```python
from build123d import *

# Parameters (mm, degrees)
CROQUIS1_R              = 1.75
SALIENTE_EXTRUIR1_DEPTH = 3


with BuildPart() as part:
    # Croquis1 → Saliente-Extruir1 (new body)
    with BuildSketch(Plane.XY):
        with BuildLine():
            Line((13.871153062, 23.274726508), (24.330135763, 23.274726508))
            ThreePointArc((24.330135763, 23.274726508), (24.799781514, 23.311715731), (25.257846044, 23.421771263))
            Line((25.257846044, 23.421771263), (32.405644412, 25.746057998))
            ThreePointArc((32.405644412, 25.746057998), (34.336780797, 30.811489821), (28.935644412, 30.347148308))
            Line((28.935644412, 30.347148308), (23.249258293, 28.345004197))
            ThreePointArc((23.249258293, 28.345004197), (22.758316719, 28.21760232), (22.252929212, 28.174726508))
            Line((22.252929212, 28.174726508), (15.948359613, 28.174726508))
            ThreePointArc((15.948359613, 28.174726508), (15.442972106, 28.21760232), (14.952030531, 28.345004197))
            Line((14.952030531, 28.345004197), (9.265644412, 30.347148308))
            ThreePointArc((9.265644412, 30.347148308), (3.864508027, 30.811489821), (5.795644412, 25.746057998))
            Line((5.795644412, 25.746057998), (12.94344278, 23.421771263))
            ThreePointArc((12.94344278, 23.421771263), (13.401507311, 23.311715731), (13.871153062, 23.274726508))
        make_face()
        with Locations((31.781902577, 28.88467969)):
            Circle(CROQUIS1_R, mode=Mode.SUBTRACT)
        with Locations(Location((6.419386247, 28.88467969, 0), (0, 0, 180))):
            Circle(CROQUIS1_R, mode=Mode.SUBTRACT)
    extrude(amount=SALIENTE_EXTRUIR1_DEPTH)


solid = part.part
```
The listing builds one solid part. Answer for the finished solid, in the listing's coordinates (mm). A direction names the side the tool comes from. Give positions to 0.01 mm unless a question says otherwise; leave off trailing zeros. Order: outer loops, then holes, each group sorted by start corner. A loop starts at its lowest first (then second) coordinate and runs counter-clockwise, first axis right, second up. Notation, with made-up numbers: (57.5, 75) - (82.5, 75) arc R17 ccw to (82.5, 88) - close; hole circle Ø5 at (87, 73). An arc over 180 degrees is marked (long way). Answer in a Markdown table with one row per item. Add a question column.
Q1. The part is cut by section D-D (x = 17). Determine the outline of the cut face in (y, z).
Q2. The part is cut by section A-A (x = 32). Determine the outline of the cut face in (y, z), then the cut area to 3 significant figures.
Q3. Find the intervals of material crossed by line 1 along X through (y, z) = (27.75, 2.05); line 2 along X through (y, z) = (28, 0.8); line 3 along Y through (x, z) = (20.5, 0.65), in increasing order. Write a range as [from, to].
Q4. Given P1, Ø1, axis at x = 20, y = 30, coming from the +Z side; P2, Ø1.5, axis at x = 17.5, z = 2, coming from the +Y side, each flat-ended and moving along its own axis, determine where each tip first touches the part or whether it passes through.
Q5. The part is cut by section B-B (y = 30). Determine the outline of the cut face in (x, z).
Q6. The part is cut by section C-C (z = 1.1). Determine the outline of the cut face in (x, y) (3 decimals).
Q7. Which of the six approach directions +Z, -Z, +X, -X, +Y, -Y give full straight-line access (tool end or side, diameter ignored) to faces 5 (the flat face through (26.13, 29.36, 1.48)), 6 (the cylindrical face through (34.39, 30.74, 1.48))?
Q8. For a pull along Y with two mould halves and no side action, classify faces 1 (the cylindrical face through (30.492, 30.067, 1.479)), 2 (the cylindrical face through (22.77, 28.22, 1.48)), 3 (the cylindrical face through (6.65, 27.15, 1.48)), 4 (the flat face through (9.32, 24.6, 1.48)) as released by +Y, released by -Y, zero draft, split by the parting line, or undercut.
Determined:
| question | item | result |
|---|---|---|
| 1 | outline | (23.27, 0) - (28.17, 0) - (28.17, 3) - (23.27, 3) - close |
| 2 | outline | (25.61, 0) - (27.15, 0) - (27.15, 3) - (25.61, 3) - close; (30.62, 0) - (32.08, 0) - (32.08, 3) - (30.62, 3) - close |
| 2 | area | 8.97 mm² |
| 3 | line 1 | x = [3.43, 5.09], [7.75, 30.45], [33.11, 34.77] |
| 3 | line 2 | x = [3.34, 4.91], [7.93, 30.27], [33.29, 34.86] |
| 3 | line 3 | y = [23.27, 28.17] |
| 4 | P1 | passes through |
| 4 | P2 | stops at y = 28.17 |
| 5 | outline | (3.42, 0) - (5.07, 0) - (5.07, 3) - (3.42, 3) - close; (7.77, 0) - (10.25, 0) - (10.25, 3) - (7.77, 3) - close; (27.95, 0) - (30.43, 0) - (30.43, 3) - (27.95, 3) - close; (33.13, 0) - (34.78, 0) - (34.78, 3) - (33.13, 3) - close |
| 6 | outline | (5.796, 25.746) - (12.943, 23.422) arc R3 ccw to (13.871, 23.275) - (24.33, 23.275) arc R3 ccw to (25.258, 23.422) - (32.406, 25.746) arc R3.2 ccw (long way) to (28.936, 30.347) - (23.249, 28.345) arc R3 cw to (22.253, 28.175) - (15.948, 28.175) arc R3 cw to (14.952, 28.345) - (9.266, 30.347) arc R3.2 ccw (long way) to start; hole circle Ø3.5 at (6.419, 28.885); hole circle Ø3.5 at (31.782, 28.885) |
| 7 | face 5 | +Z, -Z, +Y |
| 7 | face 6 | +Z, -Z |
| 8 | face 1 | undercut |
| 8 | face 2 | released by +Y |
| 8 | face 3 | undercut |
| 8 | face 4 | released by -Y |
